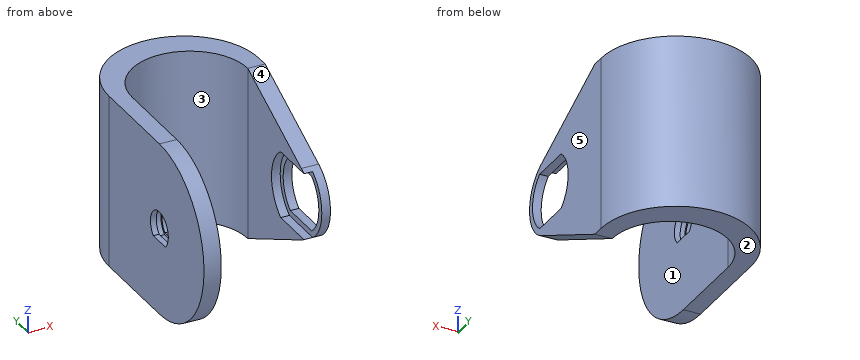
```python
from build123d import *

# Parameters (mm, degrees)
EXTRUDE_BODY_DEPTH       = 37.5
EXTRCUT_BEVELS_DEPTH     = 93.837223138
EXTRCUT_ROUNDBEVEL_DEPTH = 93.837223138
CUT_EXTRUDE13_DEPTH      = 3.75
CUT_EXTRUDE14_REACH      = 94.837
CUT_EXTRUDE15_REACH      = 99.66
CUT_EXTRUDE16_DEPTH      = 1.25


with BuildPart() as part:
    # Sketch3 → Extrude_Body (new, symmetric)
    with BuildSketch(Plane.XY):
        with BuildLine():
            Line((-25, 25), (-25, -50))
            Line((-25, -50), (-32.5, -50))
            Line((-32.5, -50), (-32.5, 30))
            ThreePointArc((-32.5, 30), (0, 62.5), (32.5, 30))
            Line((32.5, 30), (32.5, -50))
            Line((32.5, -50), (25, -50))
            Line((25, -50), (25, 25))
            ThreePointArc((25, 25), (0, 50), (-25, 25))
        make_face()
    extrude(amount=EXTRUDE_BODY_DEPTH, both=True)

    # Sketch4 → ExtrCut_Bevels (cut, through all)
    with BuildSketch(Plane.ZY.offset(-25)):
        with BuildLine():
            Line((37.5, 25), (42.5, 25))
            Line((42.5, 25), (42.5, -55.000533297))
            Line((42.5, -55.000533297), (-42.499327473, -55.000533297))
            Line((-42.499327473, -55.000533297), (-42.499327473, 24.999466703))
            Line((-42.499327473, 24.999466703), (-37.499327473, 24.999466703))
            Line((-37.499327473, 24.999466703), (-15.764161078, -20.098506949))
            ThreePointArc((-15.764161078, -20.098506949), (0.000531023, -30.000682397), (15.76513551, -20.098367466))
            Line((15.76513551, -20.098367466), (37.5, 25))
        make_face()
    extrude(amount=-EXTRCUT_BEVELS_DEPTH, mode=Mode.SUBTRACT)

    # Sketch8 → ExtrCut_RoundBevel (cut, through all)
    with BuildSketch(Plane(origin=(-25, 0, 0), x_dir=(0, 0, -1), z_dir=(1, 0, 0))):
        with BuildLine():
            Line((-37.5, -12.5), (-42.5, -12.5))
            Line((-42.5, -12.5), (-42.5, -53.627772483))
            Line((-42.5, -53.627772483), (42.5, -53.627772483))
            Line((42.5, -53.627772483), (42.5, -12.5))
            Line((42.5, -12.5), (37.5, -12.5))
            ThreePointArc((37.5, -12.5), (0, -50), (-37.5, -12.5))
        make_face()
    extrude(amount=-EXTRCUT_ROUNDBEVEL_DEPTH, mode=Mode.SUBTRACT)

    # Sketch34 → Cut-Extrude13 (cut, symmetric)
    with BuildSketch(Plane.ZY.offset(-25)):
        with BuildLine():
            Line((-14.499546396, -2.702721459), (-14.499546396, -22.298641924))
            ThreePointArc((-14.499546396, -22.298641924), (0.000453604, -30.000682398), (14.500453604, -22.298641924))
            Line((14.500453604, -22.298641924), (14.500453604, -2.702721459))
            ThreePointArc((14.500453604, -2.702721459), (0.000453604, 4.999319015), (-14.499546396, -2.702721459))
        make_face()
    extrude(amount=CUT_EXTRUDE13_DEPTH, both=True, mode=Mode.SUBTRACT)

    # Sketch35 → Cut-Extrude14 (cut, up to next)
    with BuildSketch(Plane.ZY.offset(-25), mode=Mode.PRIVATE) as cut_extrude14_sk1:
        with BuildLine():
            Line((-11.999546396, -3.500681691), (-11.999546396, -21.500681691))
            ThreePointArc((-11.999546396, -21.500681691), (0.000453604, -27.500681691), (12.000453604, -21.500681691))
            Line((12.000453604, -21.500681691), (12.000453604, -3.500681691))
            ThreePointArc((12.000453604, -3.500681691), (0.000453604, 2.499318309), (-11.999546396, -3.500681691))
        make_face()
    cut_extrude14_tool1 = extrude(cut_extrude14_sk1.sketch, amount=-CUT_EXTRUDE14_REACH, mode=Mode.PRIVATE) & part.part
    add(cut_extrude14_tool1.solids().sort_by_distance((25, -12.500682, 0.000454))[0], mode=Mode.SUBTRACT)

    # Sketch36 → Cut-Extrude15 (cut, up to next)
    with BuildSketch(Plane.ZY.offset(32.5), mode=Mode.PRIVATE) as cut_extrude15_sk1:
        with BuildLine():
            Line((-5.5, -7.400980486), (-5.5, -17.599019514))
            ThreePointArc((-5.5, -17.599019514), (7.5, -12.5), (-5.5, -7.400980486))
        make_face()
    cut_extrude15_tool1 = extrude(cut_extrude15_sk1.sketch, amount=-CUT_EXTRUDE15_REACH, mode=Mode.PRIVATE) & part.part
    add(cut_extrude15_tool1.solids().sort_by_distance((-32.5, -12.5, 0.543202))[0], mode=Mode.SUBTRACT)

    # Sketch37 → Cut-Extrude16 (cut, symmetric)
    with BuildSketch(Plane(origin=(-28.75, 0, 0), x_dir=(0, 0, -1), z_dir=(1, 0, 0))):
        with BuildLine():
            Line((6.5, -7.022774425), (6.5, -17.977225575))
            ThreePointArc((6.5, -17.977225575), (-8.5, -12.5), (6.5, -7.022774425))
        make_face()
    extrude(amount=CUT_EXTRUDE16_DEPTH, both=True, mode=Mode.SUBTRACT)


solid = part.part
```
Geometry check sheet. Reference: the model listing, model coordinates, mm. Face numbers are marked on the shaded views. A direction names the side the tool comes from. Round coordinates to 2 decimals unless told otherwise and drop trailing zeros. Loops run counter-clockwise (first coordinate to the right, second up) from the corner with the lowest first, then second, coordinate; pieces in that order, holes last. Notation, with made-up numbers: (79.25, 8) - (102.25, 8) arc R23 ccw to (102.25, 31) - close; hole circle Ø5 at (10.5, 65.5). An arc over 180 degrees is marked (long way). Write each question's results on one line, items separated by ' | '. Start each with the question number.
Q1. Thickness scan on line 1 (X direction, y = 8, z = -3); line 2 (Z direction, x = -28, y = -12); line 3 (X direction, y = -28.5, z = -8.5). Record the ranges inside material, lowest first. Write a range as [from, to].
Q2. Cross-section at B-B on y = -10. Enter the section's corners in (x, z), and give its area (3 significant figures).
Q3. Release check for a two-part mould opening along X. For the marked faces 3, 4 and 5 record: +X half, -X half, draft (parallel to the pull), parting line (faces both ways), or undercut.
Q4. Cross-section at A-A on z = 0. Enter the section's corners in (x, y).
Q5. Gauge pin test, flat ends, axial feed: P1, Ø1.2, axis at x = -26, y = -15, coming from the +Z side; P2, Ø1.9, axis at x = 27, y = -8, coming from the +Z side; P3, Ø1.1, axis at x = 31.5, y = -15, coming from the +Z side; P4, Ø12, axis at x = 15, y = 28, coming from the +Z side. Record the tip position at first contact, or that the pin passes through.
Q6. Cross-section at D-D on y = 39.5. Enter the section's corners in (x, z).
Q7. Access from +Z, -Z, +X, -X, +Y, -Y to the whole of each face (thin tool, end or side, straight path). Record for the marked faces 1 and 2.
Q8. Cross-section at C-C on z = -8.5. Enter the section's corners in (x, y).
Answers below:
1) line 1: x = [-32.5, -25], [25, 32.5] | line 2: z = [-37.5, -6.5], [8.49, 37.5] | line 3: x = [-32.5, -25]
2) outline: (-32.5, -37.5) - (-25, -37.5) - (-25, -5.5) - (-27.5, -5.5) - (-27.5, -6.5) - (-30, -6.5) - (-30, -5.5) - (-32.5, -5.5) - close; (-32.5, 7.07) - (-30, 7.07) - (-30, 8.12) - (-27.5, 8.12) - (-27.5, 7.07) - (-25, 7.07) - (-25, 37.5) - (-32.5, 37.5) - close; (25, -20.63) - (32.5, -20.63) - (32.5, -12) - (28.75, -12) - (28.75, -14.5) - (25, -14.5) - close; (25, 14.5) - (28.75, 14.5) - (28.75, 12) - (32.5, 12) - (32.5, 20.63) - (25, 20.63) - close | area: 574 mm²
3) face 3: undercut | face 4: draft | face 5: +X half
4) outline: (-32.5, -50) - (-25, -50) - (-25, -20) - (-27.5, -20) - (-27.5, -21) - (-30, -21) - (-30, -20) - (-32.5, -20) - close; (-32.5, -5) - (-30, -5) - (-30, -4) - (-27.5, -4) - (-27.5, -5) - (-25, -5) - (-25, 25) arc R25 cw to (25, 25) - (25, 5) - (28.75, 5) - (28.75, 2.5) - (32.5, 2.5) - (32.5, 30) arc R32.5 ccw to (-32.5, 30) - close; (28.75, -30) - (32.5, -30) - (32.5, -27.5) - (28.75, -27.5) - close
5) P1: stops at z = 37.45 | P2: stops at z = 22.05 | P3: stops at z = 18.49 | P4: passes through
6) outline: (-31.08, -37.5) - (-20.37, -37.5) - (-20.37, 37.5) - (-31.08, 37.5) - close; (20.37, -37.5) - (31.08, -37.5) - (31.08, 37.5) - (20.37, 37.5) - close
7) face 1: +Z, -Z, -Y | face 2: -Z, +X, -X, +Y, -Y
8) outline: (-32.5, -49.02) - (-25, -49.02) - (-25, 25) arc R25 cw to (25, 25) - (25, 2.8) - (28.75, 2.8) - (28.75, -0.14) - (32.5, -0.14) - (32.5, 30) arc R32.5 ccw to (-32.5, 30) - close; (28.75, -27.8) - (32.5, -27.8) - (32.5, -24.86) - (28.75, -24.86) - close
